from build123d import *

# Parameters (mm, degrees)
SKETCH1_R           = 60
SKETCH1_R_2         = 12.7
SKETCH1_R_3         = 3.107194875
BOSS_EXTRUDE4_DEPTH = 1
SKETCH4_R           = 1
BOSS_EXTRUDE5_DEPTH = 3
SKETCH5_R           = 18
CUT_EXTRUDE1_DEPTH  = 3


with BuildPart() as part:
    # Sketch1 → Boss-Extrude4 (new body)
    with BuildSketch(Plane.XY):
        Circle(SKETCH1_R)
        Circle(SKETCH1_R_2, mode=Mode.SUBTRACT)
        with Locations((0, 48)):
            Circle(SKETCH1_R_3, mode=Mode.SUBTRACT)
        with Locations((33.941125497, 33.941125497)):
            Circle(SKETCH1_R_3, mode=Mode.SUBTRACT)
        with Locations((48, 0)):
            Circle(SKETCH1_R_3, mode=Mode.SUBTRACT)
        with Locations((33.941125497, -33.941125497)):
            Circle(SKETCH1_R_3, mode=Mode.SUBTRACT)
        with Locations((0, -48)):
            Circle(SKETCH1_R_3, mode=Mode.SUBTRACT)
        with Locations((-33.941125497, -33.941125497)):
            Circle(SKETCH1_R_3, mode=Mode.SUBTRACT)
        with Locations((-48, 0)):
            Circle(SKETCH1_R_3, mode=Mode.SUBTRACT)
        with Locations((-33.941125497, 33.941125497)):
            Circle(SKETCH1_R_3, mode=Mode.SUBTRACT)
    extrude(amount=BOSS_EXTRUDE4_DEPTH)

    # Sketch4 → Boss-Extrude5 (add)
    with BuildSketch(Plane.XY.offset(1)):
        with Locations((0, 21)):
            Circle(SKETCH4_R)
        with Locations((21, 0)):
            Circle(SKETCH4_R)
        with Locations((0, -21)):
            Circle(SKETCH4_R)
        with Locations((-21, 0)):
            Circle(SKETCH4_R)
    extrude(amount=BOSS_EXTRUDE5_DEPTH)

    # Sketch5 → Cut-Extrude1 (cut)
    with BuildSketch(Plane.XY.offset(1)):
        Circle(SKETCH5_R)
    extrude(amount=-CUT_EXTRUDE1_DEPTH, mode=Mode.SUBTRACT)


solid = part.part
Part model, mm, in its own coordinate system. Coordinates: 2 decimals unless noted, no trailing zeros. Order: outer loops, then holes, each group sorted by start corner. A loop starts at its lowest first (then second) coordinate and runs counter-clockwise, first axis right, second up. Notation, with made-up numbers: M 3.25,35.25 L 27.25,35.25 A13 ccw 27.25,43.25 Z; hole C 53.5,11 d1. An arc over 180 degrees is marked long. Use a Markdown table: item, result.
(1) Cut at D-D on y = 24. Write the cut outline in (x, z).
A:
| item | result |
|---|---|
| outline | M -54.99,0 L 54.99,0 L 54.99,1 L -54.99,1 Z |
(2) Cut at A-A on y = 48. Write the cut outline in (x, z), then the cut area to 3 significant figures.
A:
| item | result |
|---|---|
| outline | M -36,0 L -3.11,0 L -3.11,1 L -36,1 Z; M 3.11,0 L 36,0 L 36,1 L 3.11,1 Z |
| area | 65.8 mm^2 |
(3) Pull direction Y, two halves, no side cores. Call faces 1 (the flat face through (12, 14, 0)), 2 (the cylindrical face through (-32.507, 31.185, 0.493)), 3 (the cylindrical face through (-59.94, 2.64, 0.49)): released by +Y, released by -Y, zero draft, split by the parting line, or undercut.
A:
| item | result |
|---|---|
| face 1 | zero draft |
| face 2 | undercut |
| face 3 | split by the parting line |
(4) Probe L1, parallel to Y at x = 0, z = 0.65; L2, parallel to Z at x = -11.5, y = -29.5; L3, parallel to Y at x = 43.5, z = 0.35. List the from-to ranges inside material, lowest first.
A:
| item | result |
|---|---|
| L1 | y = -60 to -51.11, -44.89 to -18, 18 to 44.89, 51.11 to 60 |
| L2 | z = 0 to 1 |
| L3 | y = -41.32 to 41.32 |
(5) Cut at B-B on x = -5.5. Write the cut outline in (y, z).
A:
| item | result |
|---|---|
| outline | M -59.75,0 L -17.14,0 L -17.14,1 L -59.75,1 Z; M 17.14,0 L 59.75,0 L 59.75,1 L 17.14,1 Z |
(6) Flat gauge pins, fed straight in: pin 1 (6 mm diameter, centred on x = 15.5, y = 36, fed in from +Z); pin 2 (3.5 mm diameter, centred on x = 48, y = 0, fed in from -Z); pin 3 (2 mm diameter, centred on y = 25.5, z = 1.5, fed in from +X); pin 4 (10 mm diameter, centred on x = -33.94, y = 33.94, fed in from -Z). Where does each tip first touch, or does it go through?
A:
| item | result |
|---|---|
| pin 1 | stops at z = 1 |
| pin 2 | passes through |
| pin 3 | stops at x = 54.71 |
| pin 4 | stops at z = 0 |
(7) Cut at C-C on z = 2.9. Write the cut outline in (x, y).
A:
| item | result |
|---|---|
| outline | C -21,0 d2; C 0,-21 d2; C 0,21 d2; C 21,0 d2 |
